```python
from build123d import *

# Parameters (mm, degrees)
CONG_1_R                     = 3
ESQUISSE2_W                  = 28.843575133
ESQUISSE2_H                  = 77
ESQUISSE2_W_2                = 77
ESQUISSE2_H_2                = 28.843575133
ENL_V_MAT_EXTRU_2_DEPTH      = 228.556586369
ENL_V_MAT_EXTRU_3_DEPTH      = 238.604187674
ENL_V_MAT_EXTRU_4_DEPTH      = 238.604187749
ENL_V_MAT_EXTRU_4_DEPTH_BACK = 238.604187749
ESQUISSE10_W                 = 22.430726153
ESQUISSE10_H                 = 145.5
PER_AGE1_START               = 162
PER_AGE1_OUTLINE_R           = 3.25
PER_AGE1_DEPTH               = 14.5
R_P_TITION_CIRCULAIRE1_COUNT = 3


# Read off the part's stored shape, not the designer's step: Perçage1
with BuildPart() as part:
    # Esquisse1 → Révolution1 (revolve)
    with BuildSketch(Plane.XY, mode=Mode.PRIVATE) as r_volution1_sk:
        Polygon((-113, 0), (-73, 0), (-63.470588237, 162), (0, 162), (0, 180), (-85, 180), (-94.529411763, 18), (-113, 18), align=None)
    revolve(r_volution1_sk.sketch.rotate(Axis((0, 193.73208918, 0), (0, -1, 0)), 270), axis=Axis((0, 193.73208918, 0), (0, -1, 0)))

    # Congé1
    cong_1_edges = [part.edges().sort_by_distance(p)[0] for p in [
        (0, 162, -63.470588237),
        (0, 18, -94.529411763),
    ]]
    fillet(cong_1_edges, radius=CONG_1_R)

    # Esquisse2 → Enlèv. mat.-Extru.2 (cut, through all)
    with BuildSketch(Plane(origin=(0, 18, 0), x_dir=(-1, 0, 0), z_dir=(0, 1, 0))):
        with Locations((120.660904657, 0)):
            Rectangle(ESQUISSE2_W, ESQUISSE2_H)
        with Locations((0, 120.660904657)):
            Rectangle(ESQUISSE2_W_2, ESQUISSE2_H_2)
        with Locations((-120.660904657, 0)):
            Rectangle(ESQUISSE2_W, ESQUISSE2_H)
    extrude(amount=-ENL_V_MAT_EXTRU_2_DEPTH, mode=Mode.SUBTRACT)

    # Esquisse5 → Enlèvement de matière-Révolution1 (revolve, cut)
    with BuildSketch(Plane.XY, mode=Mode.PRIVATE) as enl_vement_de_mati_re_r_volution1_sk:
        Polygon((-51, 180), (-51, 176.5), (-35, 176.5), (-35, 162), (0, 162), (0, 180), align=None)
    revolve(enl_vement_de_mati_re_r_volution1_sk.sketch.rotate(Axis((0, 197.596638655, 0), (0, -1, 0)), 90), axis=Axis((0, 197.596638655, 0), (0, -1, 0)), mode=Mode.SUBTRACT)

    # Esquisse9 → Enlèv. mat.-Extru.3 (cut, through all)
    with BuildSketch(Plane.XY):
        with BuildLine():
            Line((41, 117.5), (-41, 117.5))
            ThreePointArc((-41, 117.5), (-43.828427125, 116.328427125), (-45, 113.5))
            Line((-45, 113.5), (-45, 22.5))
            ThreePointArc((-45, 22.5), (-43.828427125, 19.671572875), (-41, 18.5))
            Line((-41, 18.5), (41, 18.5))
            ThreePointArc((41, 18.5), (43.828427125, 19.671572875), (45, 22.5))
            Line((45, 22.5), (45, 113.5))
            ThreePointArc((45, 113.5), (43.828427125, 116.328427125), (41, 117.5))
        make_face()
    extrude(amount=-ENL_V_MAT_EXTRU_3_DEPTH, mode=Mode.SUBTRACT)

    # Esquisse10 → Enlèv. mat.-Extru.4 (cut, two sides: drawn at the far end of the back side and taken through both)
    with BuildSketch(Plane(origin=(0, 0, 0), x_dir=(0, 0, -1), z_dir=(1, 0, 0)).offset(-ENL_V_MAT_EXTRU_4_DEPTH_BACK)):
        with Locations((82.215363077, 91.25)):
            Rectangle(ESQUISSE10_W, ESQUISSE10_H)
    extrude(amount=ENL_V_MAT_EXTRU_4_DEPTH + ENL_V_MAT_EXTRU_4_DEPTH_BACK, mode=Mode.SUBTRACT)

    # Perçage1 outline → Perçage1 (cut)
    with BuildSketch(Plane(origin=(0, 0, 0), x_dir=(1, 0, 0), z_dir=(0, 1, 0)).offset(PER_AGE1_START)):
        with Locations((35.304789832, -24.547338245)):
            Circle(PER_AGE1_OUTLINE_R)
    per_age1 = extrude(amount=PER_AGE1_DEPTH, mode=Mode.SUBTRACT)

    # Répétition circulaire1: Perçage1 ×3 about axis
    r_p_tition_circulaire1_axis = Axis((0, 0, 0), (0, 1, 0))
    for i in range(1, R_P_TITION_CIRCULAIRE1_COUNT):
        add(per_age1.rotate(r_p_tition_circulaire1_axis, i * 360 / R_P_TITION_CIRCULAIRE1_COUNT), mode=Mode.SUBTRACT)


solid = part.part
```
Can you work these out from the model? Positions are in its coordinate system, mm. A direction names the side the tool comes from. Give positions to 0.01 mm unless a question says otherwise; leave off trailing zeros. Order: outer loops, then holes, each group sorted by start corner. A loop starts at its lowest first (then second) coordinate and runs counter-clockwise, first axis right, second up. Notation, with made-up numbers: M 70.5,81 L 83.5,81 A9 cw 83.5,98 Z; hole C 47,70 d9. An arc over 180 degrees is marked long. Write item = value, one per line. Start each with the question number.
Q1. Suppose I cut it at C-C (y = 120.5). Write out the boundary of the cut face in (x, z).
Q2. I need wall thicknesses on probe 1 along Y at (x, z) = (49.5, 10); probe 2 along Y at (x, z) = (32, -95); probe 3 along Y at (x, z) = (-18, -74). Which ranges of each line are inside material? Lowest first, please. Write a range as [from, to].
Q3. We'd pull the mould along Y, two halves only. Please class faces 4 (the flat face through (26, 162, 26)), 5 (the flat face through (-45, 69, -62)), 6 (the flat face through (1, 117.5, -68)), 7 (the flat face through (-33.3, 176.5, 12)): pulls with the +Y half, pulls with the -Y half, needs draft (parallel to the pull), parting line crosses it, or undercut.
Q4. For faces 1 (the cylindrical face through (5.106, 169.148, -39.965)), 2 (the flat face through (45, 67, -62)), 3 (the flat face through (-1, 164, -77)), which set-ups out of +Z, -Z, +X, -X, +Y, -Y let a thin tool reach every point of the face, with its end or its side?
Q5. Will these pins go through, and if not, where does the flat tip stop? pin 1 Ø24.5 at (y, z) = (70, -62.5) entering from +X; pin 2 Ø1 at (y, z) = (120.5, -41) entering from +X; pin 3 Ø6 at (y, z) = (72, -39.5) entering from +X; pin 4 Ø4 at (x, z) = (-38.91, 18.3) entering from +Y.
Q6. Suppose I cut it at B-B (y = 30.5). Write out the boundary of the cut face in (x, z), plus the area to 3 significant figures.
Q7. Suppose I cut it at D-D (y = 68). Write out the boundary of the cut face in (x, z), plus the area to 3 significant figures.
Q8. Suppose I cut it at A-A (z = 0). Write out the boundary of the cut face in (x, y), plus the area to 3 significant figures.
Check result:
q1.outline = M -52.83,-71 L 52.83,-71 A88.5 ccw long Z; hole C 0,0 d131.82
q2.probe_1 = [162, 176.5]
q2.probe_2 = [0, 18]
q2.probe_3 = [0, 18.5], [164, 180]
q3.face_4 = pulls with the -Y half
q3.face_5 = undercut
q3.face_6 = undercut
q3.face_7 = pulls with the +Y half
q4.face_1 = +Y, -Y
q4.face_2 = -Z
q4.face_3 = -Z, +X, -X
q5.pin_1 = 76.48
q5.pin_2 = 78.69
q5.pin_3 = 83.76
q5.pin_4 = through
q6.outline = M -61.29,-71 L -45,-71 L -45,-55.18 A71.21 cw long 45,-55.18 L 45,-71 L 61.29,-71 A93.79 ccw long Z
q6.area = 9,360 mm2
q7.outline = M -57.86,-71 L -45,-71 L -45,-52.31 A69 cw long 45,-52.31 L 45,-71 L 57.86,-71 A91.59 ccw long Z
q7.area = 9,110 mm2
q8.outline = M -106.24,0 L -73,0 L -63.64,159.18 A3 cw -60.64,162 L -35,162 L -35,176.5 L -51,176.5 L -51,180 L -85,180 L -94.36,20.82 A3 cw -97.36,18 L -106.24,18 Z; M 35,162 L 60.64,162 A3 cw 63.64,159.18 L 73,0 L 106.24,0 L 106.24,18 L 97.36,18 A3 cw 94.36,20.82 L 85,180 L 51,180 L 51,176.5 L 35,176.5 Z
q8.area = 9,430 mm2
